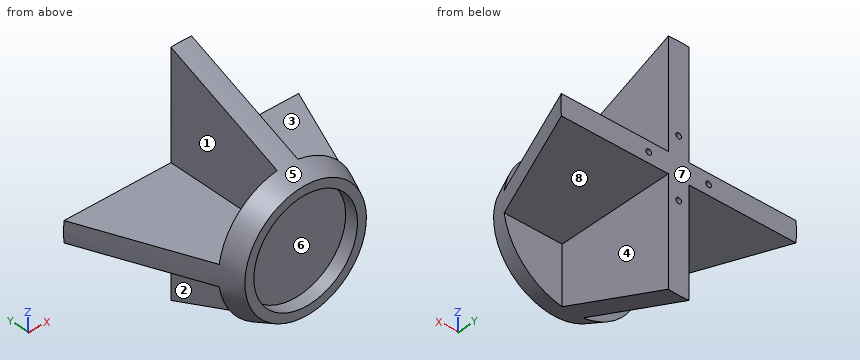
```python
from build123d import *

# Parameters (mm, degrees)
M2_5X0_45_TAPPED_HOLE1_D     = 2.05
M2_5X0_45_TAPPED_HOLE1_DEPTH = 12.7
M2_5X0_45_TAPPED_HOLE1_TIP   = 0.615882135
CROSS_WEIGHT_REDUCTION_DEPTH = 43.18
SKETCH5_R                    = 33.817028943
CUT_EXTRUDE1_DEPTH           = 0.254


with BuildPart() as part:
    # Sketch1 → Revolve1 (revolve)
    with BuildSketch(Plane(origin=(0, 0, 0), x_dir=(0, 0, -1), z_dir=(1, 0, 0))):
        Polygon((0, 0), (-19.05, 0), (-19.05, -5.08), (-22.225, -5.08), (-43.267048969, 45.72), (0, 45.72), align=None)
    revolve(axis=Axis((0, 0, 0), (0, -1, 0)))

    # M2.5x0.45 Tapped Hole1
    with Locations(Plane(origin=(0, 45.72, 0), x_dir=(1, 0, 0), z_dir=(0, 1, 0))):
        with Locations((0, 11), (11, 0), (0, -11), (-11, 0)):
            Hole(M2_5X0_45_TAPPED_HOLE1_D / 2, depth=M2_5X0_45_TAPPED_HOLE1_DEPTH)
            with Locations((0, 0, -(M2_5X0_45_TAPPED_HOLE1_DEPTH + M2_5X0_45_TAPPED_HOLE1_TIP / 2))):  # 118° drill point
                Cone(0, M2_5X0_45_TAPPED_HOLE1_D / 2, M2_5X0_45_TAPPED_HOLE1_TIP, mode=Mode.SUBTRACT)

    # Sketch2 → cross_weight_reduction (cut)
    with BuildSketch(Plane(origin=(0, 45.72, 0), x_dir=(1, 0, 0), z_dir=(0, 1, 0))):
        with BuildLine():
            Line((-3.81, -3.81), (-3.81, -43.098972452))
            ThreePointArc((-3.81, -43.098972452), (-30.594423728, -30.594423728), (-43.098972452, -3.81))
            Line((-43.098972452, -3.81), (-3.81, -3.81))
        make_face()
        with BuildLine():
            Line((-3.81, 43.098972452), (-3.81, 3.81))
            Line((-3.81, 3.81), (-43.098972452, 3.81))
            ThreePointArc((-43.098972452, 3.81), (-30.594423728, 30.594423728), (-3.81, 43.098972452))
        make_face()
        with BuildLine():
            Line((3.81, -43.098972452), (3.81, -3.81))
            Line((3.81, -3.81), (43.098972452, -3.81))
            ThreePointArc((43.098972452, -3.81), (30.594423728, -30.594423728), (3.81, -43.098972452))
        make_face()
        with BuildLine():
            Line((3.81, 3.81), (43.098972452, 3.81))
            ThreePointArc((43.098972452, 3.81), (30.594423728, 30.594423728), (3.81, 43.098972452))
            Line((3.81, 43.098972452), (3.81, 3.81))
        make_face()
    extrude(amount=-CROSS_WEIGHT_REDUCTION_DEPTH, mode=Mode.SUBTRACT)

    # Sketch5 → Cut-Extrude1 (cut)
    with BuildSketch(Plane.XZ.offset(5.08)):
        Circle(SKETCH5_R)
    extrude(amount=-CUT_EXTRUDE1_DEPTH, mode=Mode.SUBTRACT)


solid = part.part
```
Here's how the part is built. I have some questions about the finished solid (model axes, mm). Face numbers are marked on the shaded views. A direction names the side the tool comes from. Round coordinates to 2 decimals unless told otherwise and drop trailing zeros. Loops run counter-clockwise (first coordinate to the right, second up) from the corner with the lowest first, then second, coordinate; pieces in that order, holes last. Notation, with made-up numbers: (88.5, 16.5) -> (97.5, 16.5) arc R17 ccw to (97.5, 21.5) -> close; hole circle Ø1 at (-29, 71.5). An arc over 180 degrees is marked (long way). Answer as CSV lines item,"result".
1. If we section it at B-B on y = 23.5: Please give me the cut outline in (x, z).
Final values:
outline,"(-33.85, -3.81) -> (-3.81, -3.81) -> (-3.81, -33.85) arc R34.06 ccw to (3.81, -33.85) -> (3.81, -3.81) -> (33.85, -3.81) arc R34.06 ccw to (33.85, 3.81) -> (3.81, 3.81) -> (3.81, 33.85) arc R34.06 ccw to (-3.81, 33.85) -> (-3.81, 3.81) -> (-33.85, 3.81) arc R34.06 ccw to start"
2. If I drill on L1, parallel to X at y = 40, z = 11 (3 decimals); L2, parallel to Z at x = 0, y = 36.5 (3 decimals), over which ranges is the centre line in solid material (lowest first)?
Final values:
L1,"x = -3.81 to -1.025, 1.025 to 3.81"
L2,"z = -39.448 to -12.025, -9.975 to 9.975, 12.025 to 39.448"
3. Thinking about a two-plate mould opening in Z: for the marked faces 6, 7 and 8, which applies, released by +Z, released by -Z, zero draft, split by the parting line, or undercut?
Final values:
face 6,"undercut"
face 7,"zero draft"
face 8,"released by -Z"
4. If we section it at C-C on y = 7.5: Please give me the cut outline in (x, z).
Final values:
outline,"(-27.17, -3.81) -> (-3.81, -3.81) -> (-3.81, -27.17) arc R27.44 ccw to (3.81, -27.17) -> (3.81, -3.81) -> (27.17, -3.81) arc R27.44 ccw to (27.17, 3.81) -> (3.81, 3.81) -> (3.81, 27.17) arc R27.44 ccw to (-3.81, 27.17) -> (-3.81, 3.81) -> (-27.17, 3.81) arc R27.44 ccw to start"
5. If we section it at A-A on y = 35: Please give me the cut outline in (x, z) (3 decimals).
Final values:
outline,"(-38.639, -3.81) -> (-3.81, -3.81) -> (-3.81, -38.639) arc R38.827 ccw to (3.81, -38.639) -> (3.81, -3.81) -> (38.639, -3.81) arc R38.827 ccw to (38.639, 3.81) -> (3.81, 3.81) -> (3.81, 38.639) arc R38.827 ccw to (-3.81, 38.639) -> (-3.81, 3.81) -> (-38.639, 3.81) arc R38.827 ccw to start; hole circle Ø2.05 at (-11, 0); hole circle Ø2.05 at (0, -11); hole circle Ø2.05 at (0, 11); hole circle Ø2.05 at (11, 0)"
6. For pin 1 (1.6 mm diameter, centred on x = 0, z = -11, fed in from -Y); pin 2 (1 mm diameter, centred on x = 12, y = 14, fed in from +Z); pin 3 (1.5 mm diameter, centred on x = -6.5, y = 0.5, fed in from -Z), each with a flat end and sliding along its axis, tell me the tip position at first contact or that it passes through.
Final values:
pin 1,"stops at y = 0"
pin 2,"stops at z = 3.81"
pin 3,"stops at z = -24.04"
7. Which directions (+Z, -Z, +X, -X, +Y, -Y) give clear straight access to the entire face, cutting with the end or side of a thin tool? Please do the marked faces 1, 2, 3, 4 and 5.
Final values:
face 1,"+Z, -X, +Y"
face 2,"-Z, -X, +Y"
face 3,"+Z, +X, +Y"
face 4,"-Z, +X, +Y"
face 5,"-Y"
